Geometry: see drawing. Coordinates: mm, zero at the bounding-box minimum. A direction names the side the tool comes from. Give positions to 0.01 mm unless a question says otherwise; leave off trailing zeros. Order: outer loops, then holes, each group sorted by start corner. A loop starts at its lowest first (then second) coordinate and runs counter-clockwise, first axis right, second up. Notation, with made-up numbers: (68.25, 25.5) - (85.25, 25.5) arc R10 ccw to (85.25, 30.5) - close; hole circle Ø4 at (-24, 63.5). An arc over 180 degrees is marked (long way). Put each result on its own line as item: value. Start each with the question number.
1. Section C-C on z = 9.75. Return the cut outline in (x, y).
2. Section B-B on z = 19.5. Return the cut outline in (x, y), plus the area to 3 significant figures.
3. Ray query, line 1 along Z through (x, y) = (5.2, 0.8); line 2 along X through (y, z) = (1.85, 4.5); line 3 along X through (y, z) = (1.5, 2.75). Return the intervals inside material, ascending. Write a range as from..to.
4. Section D-D on y = 17. Return the cut outline in (x, z).
5. Mould query, pull axis Z, two halves, no side actions, for the marked faces 1, 2, 3 and 4. Classes: pulls with the +Z half, pulls with the -Z half, needs draft (parallel to the pull), parting line crosses it, or undercut.
6. First-contact query: P1, Ø6.5, axis at y = 19, z = 11, coming from the -X side; P2, Ø8, axis at x = 19, y = 11.5, coming from the +Z side; P3, Ø1.8, axis at y = 11.5, z = 11, coming from the +X side. Flat tips, straight axial feed; report the tip coordinate or a pass-through.
7. Section A-A on x = 36. Return the cut outline in (y, z).
8. Set-up query: the marked faces 5, 6 and 7. Return all of +Z, -Z, +X, -X, +Y, -Y with unobstructed straight access to the full face (end or side cutting, diameter ignored); none if empty.
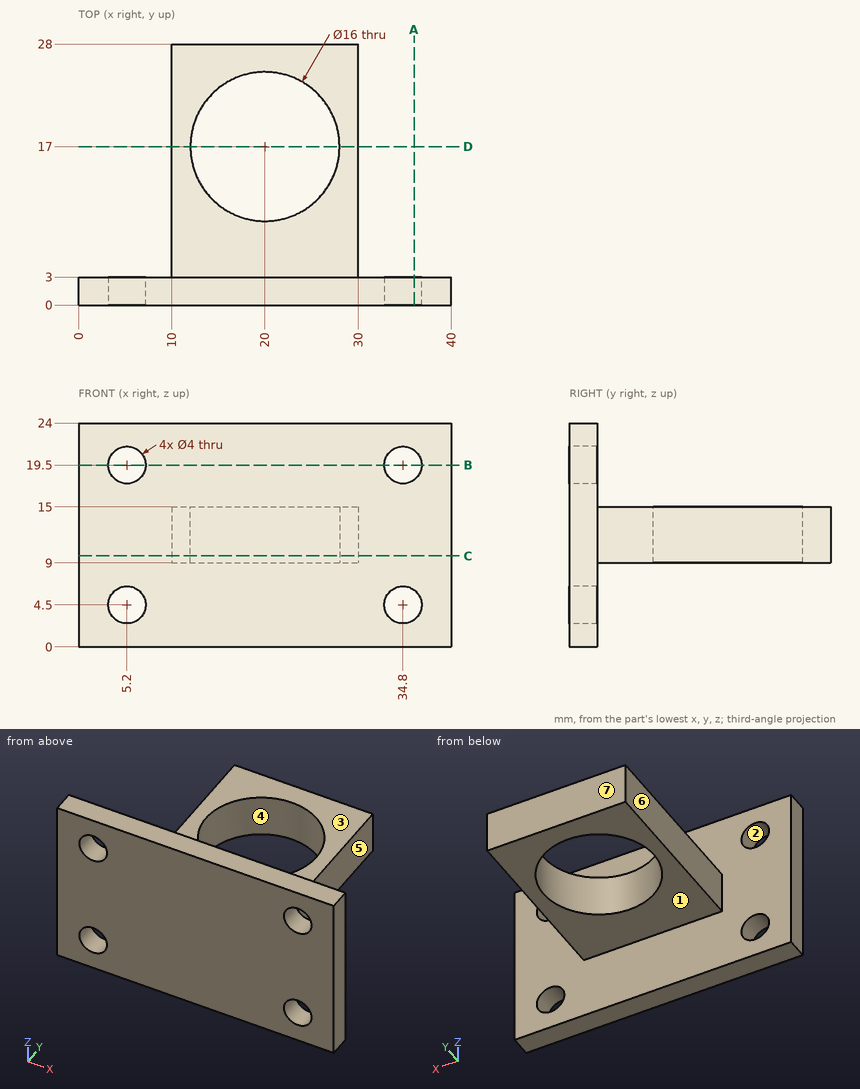
Resolved:
1. outline: (0, 0) - (40, 0) - (40, 3) - (30, 3) - (30, 28) - (10, 28) - (10, 3) - (0, 3) - close; hole circle Ø16 at (20, 17)
2. outline: (0, 0) - (3.2, 0) - (3.2, 3) - (0, 3) - close; (7.2, 0) - (32.8, 0) - (32.8, 3) - (7.2, 3) - close; (36.8, 0) - (40, 0) - (40, 3) - (36.8, 3) - close
2. area: 96.0 mm^2
3. line 1: 0..2.5, 6.5..17.5, 21.5..24
3. line 2: 0..3.2, 7.2..32.8, 36.8..40
3. line 3: 0..4.23, 6.17..33.83, 35.77..40
4. outline: (10, 9) - (12, 9) - (12, 15) - (10, 15) - close; (28, 9) - (30, 9) - (30, 15) - (28, 15) - close
5. face 1: pulls with the -Z half
5. face 2: undercut
5. face 3: pulls with the +Z half
5. face 4: needs draft
6. P1: x = 10
6. P2: z = 15
6. P3: x = 30
7. outline: (0, 0) - (3, 0) - (3, 2.9) - (0, 2.9) - close; (0, 6.1) - (3, 6.1) - (3, 17.9) - (0, 17.9) - close; (0, 21.1) - (3, 21.1) - (3, 24) - (0, 24) - close
8. face 5: +Z, -Z, +X, +Y
8. face 6: +Z, -Z, -X, +Y
8. face 7: +Z, -Z, +X, -X, +Y
